Print and shaded views of the part. All mm, measured from the part's lowest x, y and z. A direction names the side the tool comes from. Coordinates: 2 decimals unless noted, no trailing zeros. Loops run counter-clockwise (first coordinate to the right, second up) from the corner with the lowest first, then second, coordinate; pieces in that order, holes last. Notation, with made-up numbers: M 62.5,43.25 L 118.5,43.25 A14 cw 118.5,70.25 Z; hole C 57,84 d1. An arc over 180 degrees is marked long. Use a Markdown table: item, result. Add a question column.
1) Pull direction X, two halves, no side cores. Call the marked faces 4, 5 and 6: released by +X, released by -X, zero draft, split by the parting line, or undercut.
2) Wall check: probe 1 along Y at (x, z) = (11.1, 0.3); probe 2 along Y at (x, z) = (11.1, 5); probe 3 along Z at (x, y) = (19.5, 7.5). Give the ranges that are in metal, low to high. Write a range as from..to.
3) Tool access for the marked faces 1, 2 and 3: list every direction of +Z, -Z, +X, -X, +Y, -Y with a clear straight run to the whole face (end or side of a thin tool).
4) Band-saw the part on D-D (x = 16.5). List the corners of the cut face in (y, z), plus the area to 3 significant figures.
5) Band-saw the part on C-C (y = 3). List the corners of the cut face in (x, z).
6) Band-saw the part on A-A (x = 11.1). List the corners of the cut face in (y, z).
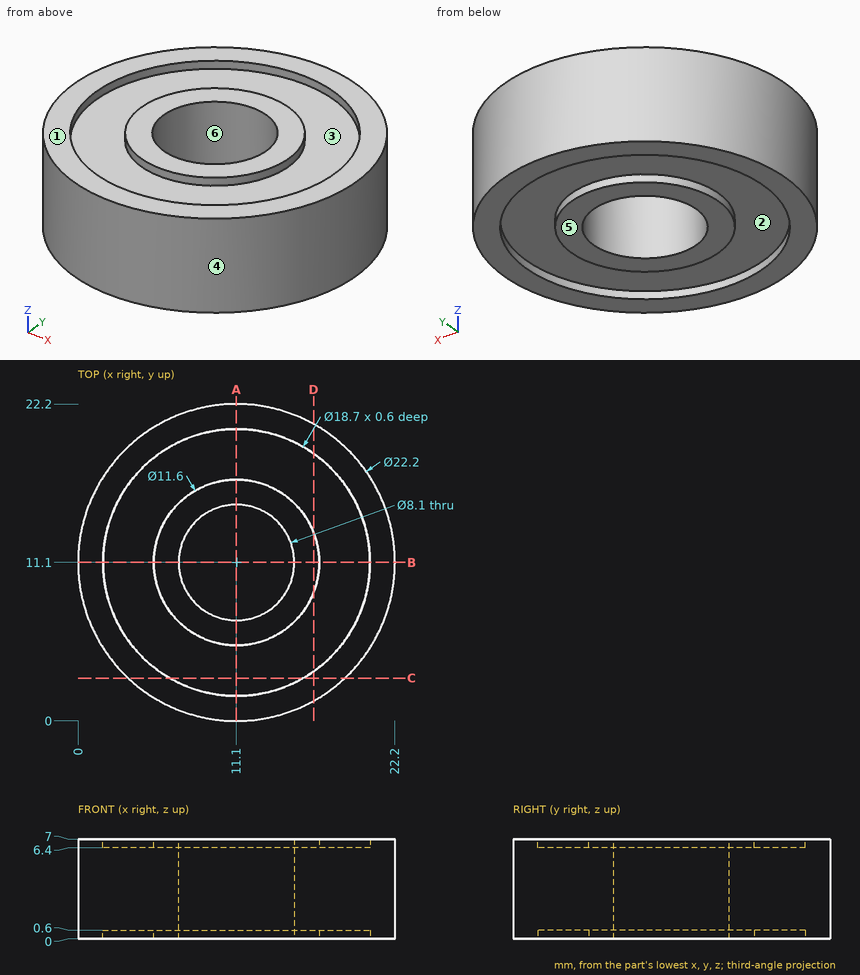
Entries:
| question | item | result |
|---|---|---|
| 1 | face 4 | split by the parting line |
| 1 | face 5 | zero draft |
| 1 | face 6 | undercut |
| 2 | probe 1 | 0..1.75, 5.3..7.05, 15.15..16.9, 20.45..22.2 |
| 2 | probe 2 | 0..7.05, 15.15..22.2 |
| 2 | probe 3 | 0.6..6.4 |
| 3 | face 1 | +Z, +X, -X, +Y, -Y |
| 3 | face 2 | -Z |
| 3 | face 3 | +Z |
| 4 | outline | M 1.4,0 L 3.47,0 L 3.47,0.6 L 8.98,0.6 L 8.98,0 L 13.22,0 L 13.22,0.6 L 18.73,0.6 L 18.73,0 L 20.8,0 L 20.8,7 L 18.73,7 L 18.73,6.4 L 13.22,6.4 L 13.22,7 L 8.98,7 L 8.98,6.4 L 3.47,6.4 L 3.47,7 L 1.4,7 Z |
| 4 | area | 123 mm2 |
| 5 | outline | M 3.51,0 L 6.43,0 L 6.43,0.6 L 15.77,0.6 L 15.77,0 L 18.69,0 L 18.69,7 L 15.77,7 L 15.77,6.4 L 6.43,6.4 L 6.43,7 L 3.51,7 Z |
| 6 | outline | M 0,0 L 1.75,0 L 1.75,0.6 L 5.3,0.6 L 5.3,0 L 7.05,0 L 7.05,7 L 5.3,7 L 5.3,6.4 L 1.75,6.4 L 1.75,7 L 0,7 Z; M 15.15,0 L 16.9,0 L 16.9,0.6 L 20.45,0.6 L 20.45,0 L 22.2,0 L 22.2,7 L 20.45,7 L 20.45,6.4 L 16.9,6.4 L 16.9,7 L 15.15,7 Z |
